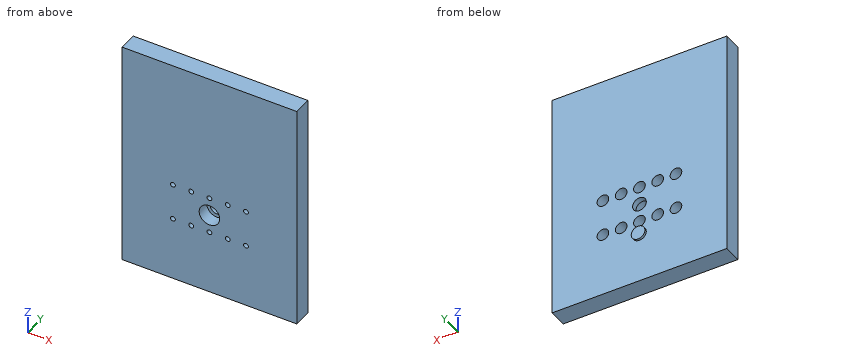
from build123d import *

# Parameters (mm, degrees)
SKETCH_1_W          = 76.6
SKETCH_1_H          = 100
SKETCH_1_R          = 3
EXTRUDE_1_DEPTH     = 8
SKETCH_2_R          = 4.5
CUT_EXTRUDE_1_DEPTH = 5.5
SKETCH_3_R          = 3
EXTRUDE_2_DEPTH     = 1
SKETCH_5_R          = 1.05
CUT_EXTRUDE_2_DEPTH = 64.489290435
SKETCH_6_R          = 2.55
CUT_EXTRUDE_3_DEPTH = 5


with BuildPart() as part:
    # ｽｹｯﾁ1 → ﾎﾞｽ - 押し出し1 (new body)
    with BuildSketch(Plane(origin=(0, 0, 0), x_dir=(1, 0, 0), z_dir=(0, 1, 0))):
        Rectangle(SKETCH_1_W, SKETCH_1_H)
        with Locations(Location((0, 14, 0), (0, 0, 270))):
            Circle(SKETCH_1_R, mode=Mode.SUBTRACT)
    extrude(amount=EXTRUDE_1_DEPTH)

    # ｽｹｯﾁ2 → ｶｯﾄ - 押し出し1 (cut)
    with BuildSketch(Plane.XZ):
        with Locations(Location((0, -14, 0), (0, 0, 270))):
            Circle(SKETCH_2_R)
    extrude(amount=-CUT_EXTRUDE_1_DEPTH, mode=Mode.SUBTRACT)

    # ｽｹｯﾁ3 → ﾎﾞｽ - 押し出し2 (add)
    with BuildSketch(Plane(origin=(0, 8, 0), x_dir=(1, 0, 0), z_dir=(0, 1, 0))):
        with Locations(Location((0, 28, 0), (0, 0, 270))):
            Circle(SKETCH_3_R)
    extrude(amount=EXTRUDE_2_DEPTH)

    # ｽｹｯﾁ5 → ｶｯﾄ - 押し出し2 (cut, through all)
    with BuildSketch(Plane(origin=(0, 8, 0), x_dir=(1, 0, 0), z_dir=(0, 1, 0))):
        with Locations(Location((0, 22, 0), (0, 0, 270))):
            Circle(SKETCH_5_R)
        with Locations(Location((8, 22, 0), (0, 0, 270))):
            Circle(SKETCH_5_R)
        with Locations(Location((16, 22, 0), (0, 0, 270))):
            Circle(SKETCH_5_R)
        with Locations(Location((-8, 22, 0), (0, 0, 270))):
            Circle(SKETCH_5_R)
        with Locations(Location((-16, 22, 0), (0, 0, 270))):
            Circle(SKETCH_5_R)
        with Locations(Location((-16, 6, 0), (0, 0, 90))):
            Circle(SKETCH_5_R)
        with Locations(Location((-8, 6, 0), (0, 0, 90))):
            Circle(SKETCH_5_R)
        with Locations(Location((16, 6, 0), (0, 0, 90))):
            Circle(SKETCH_5_R)
        with Locations(Location((8, 6, 0), (0, 0, 90))):
            Circle(SKETCH_5_R)
        with Locations(Location((0, 6, 0), (0, 0, 90))):
            Circle(SKETCH_5_R)
    extrude(amount=-CUT_EXTRUDE_2_DEPTH, mode=Mode.SUBTRACT)

    # ｽｹｯﾁ6 → ｶｯﾄ - 押し出し3 (cut)
    with BuildSketch(Plane(origin=(0, 8, 0), x_dir=(1, 0, 0), z_dir=(0, 1, 0))):
        with Locations(Location((-8, 22, 0), (0, 0, 270))):
            Circle(SKETCH_6_R)
        with Locations(Location((-16, 22, 0), (0, 0, 270))):
            Circle(SKETCH_6_R)
        with Locations(Location((0, 22, 0), (0, 0, 270))):
            Circle(SKETCH_6_R)
        with Locations(Location((8, 22, 0), (0, 0, 270))):
            Circle(SKETCH_6_R)
        with Locations(Location((16, 22, 0), (0, 0, 270))):
            Circle(SKETCH_6_R)
        with Locations(Location((-8, 6, 0), (0, 0, 270))):
            Circle(SKETCH_6_R)
        with Locations(Location((0, 6, 0), (0, 0, 270))):
            Circle(SKETCH_6_R)
        with Locations(Location((8, 6, 0), (0, 0, 270))):
            Circle(SKETCH_6_R)
        with Locations(Location((16, 6, 0), (0, 0, 270))):
            Circle(SKETCH_6_R)
        with Locations(Location((-16, 6, 0), (0, 0, 270))):
            Circle(SKETCH_6_R)
    extrude(amount=-CUT_EXTRUDE_3_DEPTH, mode=Mode.SUBTRACT)


solid = part.part
Geometry check sheet. Reference: the model listing, model coordinates, mm. Round coordinates to 2 decimals unless told otherwise and drop trailing zeros. Write each loop counter-clockwise with the first axis right and the second up, starting at its lowest first coordinate (ties: lowest second). Pieces come first, ordered by that corner, then holes. Notation, with made-up numbers: (-5, 89) -> (22, 89) arc R17 ccw to (22, 115) -> close; hole circle Ø10 at (-35.5, 30.5). An arc over 180 degrees is marked (long way). One line per item, written item: value. Start each with the question number.
(1) Cross-section at B-B, the plane x = 0. Give the number of separate pieces and of enclosed holes in the cut face, and give its area (3 significant figures).
(2) Scan lines: line 1 (X direction, y = 0.7, z = -6); line 2 (X direction, y = 6.15, z = -22); line 3 (Z direction, x = -15.5, y = 7.25). Record each from-to range of solid material in increasing order. Write a range as [from, to].
(3) Go/stop test with flat-tipped pins: pin 1 Ø4.5 at (x, z) = (8, -6) entering from +Y; pin 2 Ø1.5 at (x, z) = (28.5, 19.5) entering from +Y; pin 3 Ø4 at (x, z) = (16, -6) entering from -Y. Record where each tip stops, or that it passes through.
(4) Cross-section at A-A, the plane x = 8. Record the cut outline in (y, z), and give its area (3 significant figures).
(5) Cross-section at D-D, the plane z = -28. Record the cut outline in (x, y), and give its area (3 significant figures).
Answer:
1. separate pieces: 4
1. enclosed holes: 0
1. area: 678 mm²
2. line 1: [-38.3, -17.05], [-14.95, -9.05], [-6.95, -1.05], [1.05, 6.95], [9.05, 14.95], [17.05, 38.3]
2. line 2: [-38.3, -18.55], [-13.45, -10.55], [-5.45, -2.55], [2.55, 5.45], [10.55, 13.45], [18.55, 38.3]
2. line 3: [-50, -24.5], [-19.5, -8.5], [-3.5, 50]
3. pin 1: y = 3
3. pin 2: y = 8
3. pin 3: y = 0
4. outline: (0, -50) -> (8, -50) -> (8, -24.55) -> (3, -24.55) -> (3, -23.05) -> (0, -23.05) -> close; (0, -20.95) -> (3, -20.95) -> (3, -19.45) -> (8, -19.45) -> (8, -8.55) -> (3, -8.55) -> (3, -7.05) -> (0, -7.05) -> close; (0, -4.95) -> (3, -4.95) -> (3, -3.45) -> (8, -3.45) -> (8, 50) -> (0, 50) -> close
4. area: 736 mm²
5. outline: (-38.3, 0) -> (38.3, 0) -> (38.3, 8) -> (3, 8) -> (3, 9) -> (-3, 9) -> (-3, 8) -> (-38.3, 8) -> close
5. area: 619 mm²
